For this review, take the finished solid that the model builds, in its own axes (mm). A direction names the side the tool comes from. Give positions to 0.01 mm unless a question says otherwise; leave off trailing zeros. Loops run counter-clockwise (first coordinate to the right, second up) from the corner with the lowest first, then second, coordinate; pieces in that order, holes last. Notation, with made-up numbers: (-28.5, 18) - (22.5, 18) arc R31 ccw to (22.5, 44) - close; hole circle Ø10 at (69, 50.5). An arc over 180 degrees is marked (long way). Answer in a Markdown table with one row per item.
Autodesk Inventor part; units mm, degrees
ref_plane "YZ Plane" through (0, 0, 0) normal (1, 0, 0) x (0, 1, 0)
ref_plane "XZ Plane" through (0, 0, 0) normal (0, 1, 0) x (-1, 0, 0)
ref_plane "XY Plane" through (0, 0, 0) normal (0, 0, 1) x (1, 0, 0)
sketch "Boceto1" plane through (0, 0, 0) normal (0, 1, 0) x (-1, 0, 0)
  line L0 (3, 0) -> (33, 0)
  line L1 (36, -3) -> (36, -62)
  line L2 (33, -65) -> (3, -65)
  line L3 (0, -62) -> (0, -3)
  circle A0 centre (3.5, -61.5) radius 1.375
  arc A1 (36, -3) -> (33, 0) centre (33, -3) ccw
  arc A2 (3, 0) -> (0, -3) centre (3, -3) ccw
  arc A3 (0, -62) -> (3, -65) centre (3, -62) ccw
  arc A4 (33, -65) -> (36, -62) centre (33, -62) ccw
  circle A5 centre (26.5, -61.5) radius 1.375
  circle A6 centre (3.5, -3.5) radius 1.375
  circle A7 centre (26.5, -3.5) radius 1.375
  line L4 (36, 0) -> (0, 0)
  line L5 (0, 0) -> (0, 10)
  line L6 (0, 10) -> (36, 10)
  line L7 (36, 10) -> (36, 0)
  line L8 (36, -65) -> (0, -65)
  line L9 (0, -65) -> (0, -75)
  line L10 (0, -75) -> (36, -75)
  line L11 (36, -75) -> (36, -65)
  line L12 (7.5, 0) -> (20.5, 0)
  line L13 (20.5, 0) -> (20.5, 10)
  line L14 (20.5, 10) -> (7.5, 10)
  line L15 (7.5, 10) -> (7.5, 0)
  line L16 (7.5, 0) -> (20.5, 10) construction
  line L17 (20.5, 0) -> (7.5, 10) construction
  line L18 (7.5, -75) -> (20.5, -75)
  line L19 (20.5, -75) -> (20.5, -65)
  line L20 (20.5, -65) -> (7.5, -65)
  line L21 (7.5, -65) -> (7.5, -75)
  line L22 (7.5, -75) -> (20.5, -65) construction
  line L23 (20.5, -75) -> (7.5, -65) construction
  line L24 (36, -32.5) -> (0, -32.5)
  line L25 (36, 0) -> (36, -3)
  line L26 (0, 0) -> (0, -3)
  line L27 (0, -62) -> (0, -65)
  line L28 (36, -62) -> (36, -65)
  line L29 (36, -22.5) -> (49, -22.5)
  line L30 (49, -22.5) -> (49, -42.5)
  line L31 (49, -42.5) -> (36, -42.5)
  line L32 (36, -42.5) -> (36, -22.5)
  arc A8 (49, -42.5) -> (49, -22.5) centre (49, -32.5) ccw
  line L33 (20.5, 5.3) -> (23.5, 5.3)
  line L34 (23.5, 5.3) -> (23.5, 3)
  line L35 (23.5, 3) -> (20.5, 3)
  line L36 (20.5, 3) -> (20.5, 5.3)
  arc A9 (23.5, 3) -> (23.5, 5.3) centre (23.5, 4.15) ccw
  line L37 (14, 0) -> (14, -65)
  line L38 (7.5, 5.3) -> (4.5, 5.3)
  line L39 (4.5, 5.3) -> (4.5, 3)
  line L40 (4.5, 3) -> (7.5, 3)
  line L41 (7.5, 3) -> (7.5, 5.3)
  arc A10 (4.5, 5.3) -> (4.5, 3) centre (4.5, 4.15) ccw
  line L42 (20.5, -70.3) -> (23.5, -70.3)
  line L43 (23.5, -70.3) -> (23.5, -68)
  line L44 (23.5, -68) -> (20.5, -68)
  line L45 (20.5, -68) -> (20.5, -70.3)
  arc A11 (23.5, -70.3) -> (23.5, -68) centre (23.5, -69.15) ccw
  line L46 (4.5, -68) -> (7.5, -68)
  arc A12 (4.5, -68) -> (4.5, -70.3) centre (4.5, -69.15) ccw
  line L47 (7.5, -70.3) -> (4.5, -70.3)
  line L48 (4.5, -70.3) -> (4.5, -68)
  line L49 (7.5, -68) -> (7.5, -70.3)
  line L50 (36, 0) -> (49, 0)
  line L51 (49, 0) -> (49, -65)
  line L52 (49, -65) -> (36, -65)
  line L53 (36, -65) -> (36, 0)
  line L54 (44, -20) -> (41, -20)
  line L55 (41, -20) -> (41, -45)
  line L56 (41, -45) -> (44, -45)
  line L57 (44, -45) -> (44, -20)
  line L58 (36, 10) -> (36, 18)
  line L59 (36, -75) -> (36, -83)
  arc A13 (36, -83) -> (36, 18) centre (-7.9402, -32.5) ccw
  line L60 (0, -75) -> (-8, -75)
  line L61 (-8, -75) -> (-8, 10)
  line L62 (-8, 10) -> (0, 10)
  line L63 (0, 10) -> (0, -75)
  line L64 (-8, 10) -> (-8, 17.5724)
  line L65 (-8, -75) -> (-8, -82.5724)
  arc A14 (-8, 17.5724) -> (-8, -82.5724) centre (14, -32.5) ccw
  circle A15 centre (118.6884, -49.4222) radius 60
  point P0 (14, 5)
  point P1 (14, -70)
  point P2 (36, -42.5)
  point P3 (7.5, -70.3)
  point P4 (20.5, -70.3)
  point P5 (7.5, 5.3)
  point P6 (20.5, 3)
  point P7 (44, -32.5)
  point P8 (36, -65)
  point P9 (44, -42.5)
  point P10 (41, -42.5)
  point P11 (41, -22.5)
  point P12 (44, -22.5)
  point P13 (49, -22.5)
  point P14 (59, -32.5)
  dimension "d0" = 36
  dimension "d1" = 65
  dimension "d2" = 2.75
  dimension "d3" = 3
  dimension "d4" = 3
  dimension "d5" = 3
  dimension "d6" = 3
  dimension "d7" = 3.5
  dimension "d8" = 3.5
  dimension "d11" = 23
  dimension "d14" = 58
  dimension "d17" = 10
  dimension "d18" = 10
  dimension "d19" = 13
  dimension "d20" = 10
  dimension "d21" = 13
  dimension "d22" = 10
  dimension "d26" = 7.5
  dimension "d30" = 20
  dimension "d31" = 13
  dimension "d32" = 3
  dimension "d33" = 2.3
  dimension "d34" = 3
  dimension "d35" = 1.15
  dimension "d36" = 13
  dimension "d37" = 3
  dimension "d38" = 25
  dimension "d39" = 5
  dimension "d42" = 8
  dimension "d43" = 8
  dimension "d46" = 8
  dimension "d47" = 54.6923
  dimension "d50" = 120
extrude "Extrusión1" add sketch "Boceto1" along normal blind 3 contours L4 L5 L6 L15 L38 A10 L40 L0 | L0 L37 L24 L3 A2 | A2 L26 L4 | L15 L6 L13 L0 | L0 A1 L1 L24 L37 | L24 L37 L2 A3 L3 | L13 L35 A9 L33 L6 L7 L4 L0 | L24 L1 A4 L2 L37 | A3 L8 L27 | L4 L25 A1 | L1 L29 L55 L31 | L2 L19 L10 L21 | L2 L21 L46 A12 L47 L10 L9 L8 | L25 L50 L51 L29 L57 L54 L55 L1 | L7 L58 A13 A8 L51 L50 | L31 L55 L56 L57 L51 L52 L28 L1 | L2 L8 L11 L10 L19 L42 A11 L44 | L29 L57 L31 L55 | L28 L8 A4 | L30 L31 L57 L29 | A8 L30 | L52 L51 A8 A13 L59 L11
fillet "Empalme1" radius 10 2 edges at (0, 1.5, -75) (0, 1.5, 10)
extrude "Extrusión2" cut sketch "Boceto1" along normal blind 3 contours L29 L57 L31 L55
fillet "Empalme2" radius 2 4 edges at (-36, 1.5, -83) (-36, 1.5, 18) (-36, 1.5, 10) (-36, 1.5, -75)
extrude "Extrusión3" add sketch "Boceto1" along normal blind 3 contours L4 L5 L6 L15 L38 A10 L40 L0 | L3 L27 L9 L60 L61 L62 L5 L26 | L61 L65 A14 L64 | L2 L21 L46 A12 L47 L10 L9 L8
equation "\"d18\" = d17"
equation "\"d21\" = d19"
equation "\"d22\" = d20"
equation "\"d36\" = d31"
properties part number "Parte inferior 2"
1. Wall thickness on line 1 (Z direction, x = -26.5, y = 1.25) (3 decimals); line 2 (X direction, y = 0.85, z = -34); line 3 (X direction, y = 2.05, z = -28): over which ranges is each line inside the solid? List them lowest first. Write a range as [from, to].
Values:
| item | result |
|---|---|
| line 1 | z = [-75, -62.875], [-60.125, -4.875], [-2.125, 10] |
| line 2 | x = [-58.98, -44], [-41, 40.67] |
| line 3 | x = [-58.85, -44], [-41, 40.51] |
2. We need section D-D, the plane x = 1. Give the boundary of the cut face in (y, z), and give its area (3 significant figures).
Values:
| item | result |
|---|---|
| outline | (0, -75) - (3, -75) - (3, 10) - (0, 10) - close |
| area | 255 mm^2 |
3. For faces 1 (the face through (8, 1, -79)), 2 (the face through (-22, 1, -68)), 3 (the face through (8, 1, 14)), list the 3-axis set-ups (+Z, -Z, +X, -X, +Y, -Y) from which the entire face can be reached by the end or side of a thin tool; tool diameter is ignored.
Values:
| item | result |
|---|---|
| face 1 | -Z, +Y, -Y |
| face 2 | +Y, -Y |
| face 3 | +Z, +Y, -Y |
4. We need section B-B, the plane z = -3.5. Give the boundary of the cut face in (x, y) (3 decimals), and give its area (3 significant figures).
Values:
| item | result |
|---|---|
| outline | (-52.392, 0) - (-27.875, 0) - (-27.875, 3) - (-52.392, 3) - close; (-25.125, 0) - (-4.875, 0) - (-4.875, 3) - (-25.125, 3) - close; (-2.125, 0) - (32.371, 0) - (32.371, 3) - (-2.125, 3) - close |
| area | 238 mm^2 |
5. We need section A-A, the plane x = -26.5. Give the boundary of the cut face in (y, z) (3 decimals).
Values:
| item | result |
|---|---|
| outline | (0, -75) - (3, -75) - (3, -62.875) - (0, -62.875) - close; (0, -60.125) - (3, -60.125) - (3, -4.875) - (0, -4.875) - close; (0, -2.125) - (3, -2.125) - (3, 10) - (0, 10) - close |
6. Clearance check with flat-ended pins moving along their axes: pin 1 (2.5 mm diameter, centred on x = -3.5, z = -61.5, fed in from +Y); pin 2 (0.9 mm diameter, centred on x = -6.5, y = 2, fed in from -Z); pin 3 (1.5 mm diameter, centred on y = 2, z = -14, fed in from +X); pin 4 (1.5 mm diameter, centred on x = -43, y = 2, fed in from +Z). State where each tip first meets the part, or that it passes through.
Values:
| item | result |
|---|---|
| pin 1 | passes through |
| pin 2 | stops at z = -75 |
| pin 3 | stops at x = 37.73 |
| pin 4 | stops at z = 11.79 |
7. We need section C-C, the plane y = 1.85. Count the separate pieces of the cut face and the enclosed holes in it, and give its area (3 significant figures).
Values:
| item | result |
|---|---|
| separate pieces | 1 |
| enclosed holes | 9 |
| area | 7,570 mm^2 |
8. Mouldability with a two-part tool opening along Z and no side actions: class faces 4 (the face through (-37.27, 1.52, 15.26)), 5 (the face through (-24.65, 1.48, -69.12)), 6 (the face through (-20.5, 1, -69)), 7 (the face through (-22, 1, -75)) as released by +Z, released by -Z, zero draft, split by the parting line, or undercut.
Values:
| item | result |
|---|---|
| face 4 | released by +Z |
| face 5 | undercut |
| face 6 | undercut |
| face 7 | released by -Z |
